Geometry check sheet. Reference: the model listing, model coordinates, mm. Round coordinates to 2 decimals unless told otherwise and drop trailing zeros. Write each loop counter-clockwise with the first axis right and the second up, starting at its lowest first coordinate (ties: lowest second). Pieces come first, ordered by that corner, then holes. Notation, with made-up numbers: (41.5, 58.5) -> (100.5, 58.5) arc R34 ccw to (100.5, 95.5) -> close; hole circle Ø11 at (54, -3). An arc over 180 degrees is marked (long way). Return JSON: item names as keys, results as strings. Group by question number.
from build123d import *

# Parameters (mm, degrees)
CROQUIS4_W              = 40
CROQUIS4_H              = 84
SALIENTE_EXTRUIR3_DEPTH = 5
CROQUIS5_R              = 7
CORTAR_EXTRUIR1_DEPTH   = 5
CROQUIS5_3_R            = 7
CORTAR_EXTRUIR2_DEPTH   = 5


with BuildPart() as part:
    # Croquis4 → Saliente-Extruir3 (new body)
    with BuildSketch(Plane.XY):
        with Locations((20, 42)):
            Rectangle(CROQUIS4_W, CROQUIS4_H)
    extrude(amount=SALIENTE_EXTRUIR3_DEPTH)

    # Croquis5 → Cortar-Extruir1 (cut)
    with BuildSketch(Plane.XY.offset(5)):
        with Locations((20, 63)):
            Circle(CROQUIS5_R)
    extrude(amount=-CORTAR_EXTRUIR1_DEPTH, mode=Mode.SUBTRACT)

    # Croquis5<3> → Cortar-Extruir2 (cut)
    with BuildSketch(Plane.XY.offset(5)):
        with Locations((20, 21)):
            Circle(CROQUIS5_3_R)
    extrude(amount=-CORTAR_EXTRUIR2_DEPTH, mode=Mode.SUBTRACT)


solid = part.part
1) Sectioned sample at A-A on x = 20. Enter the section's corners in (y, z), and give its area (3 significant figures).
2) Mould release check, pull along X, two halves, no side actions. Record for faces 1 (the face through (19.09, 69.94, 2.54)), 2 (the face through (0, 41, 2)), 3 (the face through (40, 41, 2)), 4 (the face through (20, 43, 5)): +X half, -X half, draft (parallel to the pull), parting line (faces both ways), or undercut.
3) Material ranges on probe 1 along Y at (x, z) = (20, 3.15); probe 2 along Y at (x, z) = (22, 2.5); probe 3 along X at (y, z) = (22.5, 1.8), recorded low to high. Write a range as [from, to].
4) Sectioned sample at C-C on z = 1.8. Enter the section's corners in (x, y).
5) Sectioned sample at B-B on y = 63. Enter the section's corners in (x, z).
6) Go/stop test with a flat-tipped pin: P1, Ø3, axis at x = 8.5, z = 1, coming from the -Y side. Record where the tip stops, or that it passes through.
Evaluation:
{
 "1": {"outline": "(0, 0) -> (14, 0) -> (14, 5) -> (0, 5) -> close; (28, 0) -> (56, 0) -> (56, 5) -> (28, 5) -> close; (70, 0) -> (84, 0) -> (84, 5) -> (70, 5) -> close", "area": "280 mm2"},
 "2": {"face 1": "undercut", "face 2": "-X half", "face 3": "+X half", "face 4": "draft"},
 "3": {"probe 1": "y = [0, 14], [28, 56], [70, 84]", "probe 2": "y = [0, 14.29], [27.71, 56.29], [69.71, 84]", "probe 3": "x = [0, 13.16], [26.84, 40]"},
 "4": {"outline": "(0, 0) -> (40, 0) -> (40, 84) -> (0, 84) -> close; hole circle Ø14 at (20, 21); hole circle Ø14 at (20, 63)"},
 "5": {"outline": "(0, 0) -> (13, 0) -> (13, 5) -> (0, 5) -> close; (27, 0) -> (40, 0) -> (40, 5) -> (27, 5) -> close"},
 "6": {"P1": "stops at y = 0"}
}
